Here's the drawing with two shaded views (mm, measured from the low corner). I have some questions. A direction names the side the tool comes from. Round coordinates to 2 decimals unless told otherwise and drop trailing zeros. Loops run counter-clockwise (first coordinate to the right, second up) from the corner with the lowest first, then second, coordinate; pieces in that order, holes last. Notation, with made-up numbers: (46, 56) -> (51, 56) arc R14 ccw to (51, 76) -> close; hole circle Ø2 at (81, 11). An arc over 180 degrees is marked (long way). Write each question's results on one line, items separated by ' | '. Start each with the question number.
1) We'd pull the mould along X, two halves only. Please class the marked faces 1, 2, 3 and 4: pulls with the +X half, pulls with the -X half, needs draft (parallel to the pull), parting line crosses it, or undercut.
2) Imagine slicing it at D-D, the plane y = 24.5. List the corners of the cut face in (x, z) for me.
3) Imagine slicing it at A-A, the plane x = 12.5. List the corners of the cut face in (y, z) for me.
4) Imagine slicing it at C-C, the plane y = 7.5. List the corners of the cut face in (x, z) for me, plus the area to 3 significant figures.
5) For P1, Ø4.5, axis at x = 30, y = 7.5, coming from the -Z side; P2, Ø10, axis at x = 30.5, z = 18, coming from the +Y side; P3, Ø7.5, axis at x = 29.5, z = 7.5, coming from the -Y side, each with a flat end and sliding along its axis, tell me the tip position at first contact or that it passes through.
6) Which directions (+Z, -Z, +X, -X, +Y, -Y) give clear straight access to the entire face, cutting with the end or side of a thin tool? Please do the marked faces 5, 6 and 7.
7) If I drill on probe 1 along X at (y, z) = (16, 7.5); probe 2 along Y at (x, z) = (30, 16.05); probe 3 along X at (y, z) = (22, 8.75), over which ranges is the centre line in solid material (lowest first)?
8) Imagine slicing it at B-B, the plane z = 3. List the corners of the cut face in (x, y) for me, plus the area to 3 significant figures.
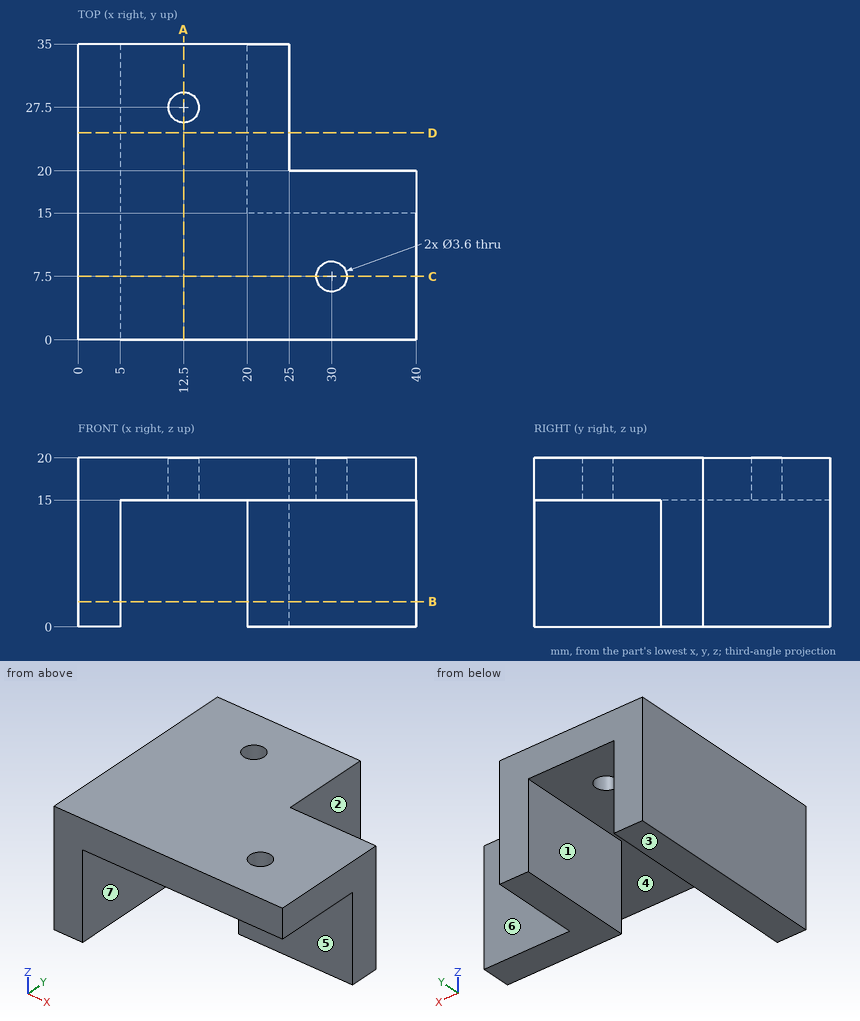
Checked values:
1) face 1: undercut | face 2: pulls with the +X half | face 3: needs draft | face 4: undercut
2) outline: (0, 0) -> (5, 0) -> (5, 15) -> (20, 15) -> (20, 0) -> (25, 0) -> (25, 20) -> (0, 20) -> close
3) outline: (0, 15) -> (25.7, 15) -> (25.7, 20) -> (0, 20) -> close; (29.3, 15) -> (35, 15) -> (35, 20) -> (29.3, 20) -> close
4) outline: (0, 0) -> (5, 0) -> (5, 15) -> (28.2, 15) -> (28.2, 20) -> (0, 20) -> close; (31.8, 15) -> (40, 15) -> (40, 20) -> (31.8, 20) -> close | area: 257 mm^2
5) P1: z = 15 | P2: y = 20 | P3: y = 15
6) face 5: -Z, +X, -Y | face 6: +Z, -Z, +X, +Y | face 7: -Z, +Y, -Y
7) probe 1: 0 to 5, 20 to 40 | probe 2: 0 to 5.7, 9.3 to 20 | probe 3: 0 to 5, 20 to 25
8) outline: (0, 0) -> (5, 0) -> (5, 35) -> (0, 35) -> close; (20, 15) -> (40, 15) -> (40, 20) -> (25, 20) -> (25, 35) -> (20, 35) -> close | area: 350 mm^2
